Read the model definition and answer for the solid it produces. Units are mm, in the model's axes. A direction names the side the tool comes from. Give positions to 0.01 mm unless a question says otherwise; leave off trailing zeros. Loops run counter-clockwise (first coordinate to the right, second up) from the corner with the lowest first, then second, coordinate; pieces in that order, holes last. Notation, with made-up numbers: (-31, 1) -> (27, 1) arc R22 ccw to (27, 21) -> close; hole circle Ø9 at (-33.5, 20). An arc over 180 degrees is marked (long way). Write each question's results on one line, items separated by ' | '. Start each with the question number.
Item 1: Each of these flat-tipped pins is pushed along its axis until it touches: P1, Ø4, axis at y = -3, z = 19, coming from the -X side; P2, Ø5, axis at x = 2.5, y = 1.5, coming from the -Z side; P3, Ø3, axis at y = 0.5, z = 14.5, coming from the -X side; P4, Ø1, axis at y = 3, z = 11.5, coming from the +X side. Where does it stop, or does it pass through?
Item 2: Which of the six approach directions +Z, -Z, +X, -X, +Y, -Y give full straight-line access (tool end or side, diameter ignored) to faces 4 (the flat face through (-2, -2, 7.075)), 5 (the cylindrical face through (3, 0, 14)), 6 (the cylindrical face through (5.994, -0.264, 21.368))?
Item 3: Section D-D on z = 19 is taken. Write down the section's boundary in (x, y), and give its area (3 significant figures).
Item 4: Determine the mould class of faces 1 (the flat face through (2, -2, 7.875)), 2 (the cylindrical face through (3, -0.1, 6.5)), 3 (the flat face through (3, 1, 20.875)) for opening direction Z: +Z half, -Z half, draft (parallel to the pull), parting line (faces both ways), or undercut.
Item 5: Section A-A on y = 0 is taken. Write down the section's boundary in (x, z), and give its area (3 significant figures).
Item 6: Section C-C on z = 21.5 is taken. Write down the section's boundary in (x, y), and give its area (3 significant figures).
Item 7: Find the intervals of material crossed by line 1 (Z direction, x = -2, y = 3.25); line 2 (X direction, y = 1.25, z = 15.25); line 3 (Z direction, x = 4.25, y = -4), in increasing order.
```python
from build123d import *

# Parameters (mm, degrees)
CHAMFER1_SIZE = 0.5


with BuildPart() as part:
    # Sketch1 → Revolve1 (revolve)
    with BuildSketch(Plane(origin=(0, 0, 0), x_dir=(1, 0, 0), z_dir=(0, 1, 0))):
        Polygon((0, -22.374712644), (-6, -22.374712644), (-6, -20.874712644), (-3, -20.874712644), (-3, -7.874712644), (-2.5, -7.874712644), (-2.5, -7.074712644), (-3, -7.074712644), (-3, -5.374712644), (0, -5.374712644), align=None)
    revolve(axis=Axis((0, 0, -21.276149425), (0, 0, 1)))

    # Chamfer1
    chamfer1_edges = [part.edges().sort_by_distance(p)[0] for p in [
        (3, 0, 5.374712644),
        (6, 0, 22.374712644),
    ]]
    chamfer(chamfer1_edges, length=CHAMFER1_SIZE)


solid = part.part
```
Findings:
1) P1: x = -5.54 | P2: z = 5.37 | P3: x = -3 | P4: x = 1.66
2) face 4: none | face 5: -Z | face 6: +Z, -Z
3) outline: circle Ø6 at (0, 0) | area: 28.3 mm2
4) face 1: undercut | face 2: draft | face 3: -Z half
5) outline: (-6, 20.87) -> (-3, 20.87) -> (-3, 7.87) -> (-2.5, 7.87) -> (-2.5, 7.07) -> (-3, 7.07) -> (-3, 5.87) -> (-2.5, 5.37) -> (2.5, 5.37) -> (3, 5.87) -> (3, 7.07) -> (2.5, 7.07) -> (2.5, 7.87) -> (3, 7.87) -> (3, 20.87) -> (6, 20.87) -> (6, 21.87) -> (5.5, 22.37) -> (-5.5, 22.37) -> (-6, 21.87) -> close | area: 110 mm2
6) outline: circle Ø12 at (0, 0) | area: 113 mm2
7) line 1: 20.87 to 22.37 | line 2: -2.73 to 2.73 | line 3: 20.87 to 22.04
